Work out the finished part from the listing and answer in its coordinate system (mm). A direction names the side the tool comes from. Round coordinates to 2 decimals unless told otherwise and drop trailing zeros. Loops run counter-clockwise (first coordinate to the right, second up) from the corner with the lowest first, then second, coordinate; pieces in that order, holes last. Notation, with made-up numbers: (86.5, 5.25) -> (139.5, 5.25) arc R21 ccw to (139.5, 29.25) -> close; hole circle Ø6 at (-15, 56.5). An arc over 180 degrees is marked (long way). Use one line per item in the form item = value.
```python
from build123d import *

# Parameters (mm, degrees)
SKETCH_1_W          = 50
SKETCH_1_H          = 150
EXTRUDE_1_DEPTH     = 40
CHAMFER_1_SIZE      = 30
CHAMFER_1_SIZE2     = 60
FILLET_1_R          = 10
SKETCH_2_R          = 10
CUT_EXTRUDE_1_DEPTH = 15
CHAMFER_2_SIZE      = 1
SKETCH_3_R          = 5
CUT_EXTRUDE_2_DEPTH = 26


with BuildPart() as part:
    # 草图1 → 凸台-拉伸1 (new body)
    with BuildSketch(Plane.XY):
        with Locations((25, 75)):
            Rectangle(SKETCH_1_W, SKETCH_1_H)
    extrude(amount=EXTRUDE_1_DEPTH)

    # 倒角1
    chamfer_1_edges = [part.edges().sort_by_distance(p)[0] for p in [
        (25, 0, 40),
    ]]
    chamfer_1_side = [part.faces().sort_by_distance(p)[0] for p in [
        (25, 0, 20),
    ]]
    chamfer(chamfer_1_edges, length=CHAMFER_1_SIZE, length2=CHAMFER_1_SIZE2, reference=chamfer_1_side[0])

    # 圆角1
    fillet_1_edges = [part.edges().sort_by_distance(p)[0] for p in [
        (25, 60, 40),
    ]]
    fillet(fillet_1_edges, radius=FILLET_1_R)

    # 草图2 → 切除-拉伸1 (cut)
    with BuildSketch(Plane.XY.offset(40)):
        with Locations((25, 130)):
            Circle(SKETCH_2_R)
        with Locations((25, 80)):
            Circle(SKETCH_2_R)
    extrude(amount=-CUT_EXTRUDE_1_DEPTH, mode=Mode.SUBTRACT)

    # 倒角2
    chamfer_2_edges = [part.edges().sort_by_distance(p)[0] for p in [
        (15, 130, 40),
        (15, 80, 40),
    ]]
    chamfer(chamfer_2_edges, length=CHAMFER_2_SIZE)

    # 草图3 → 切除-拉伸2 (cut, through all)
    with BuildSketch(Plane.XY.offset(25)):
        with Locations((25, 130)):
            Circle(SKETCH_3_R)
        with Locations((25, 80)):
            Circle(SKETCH_3_R)
    extrude(amount=-CUT_EXTRUDE_2_DEPTH, mode=Mode.SUBTRACT)


solid = part.part
```
(1) Given P1, Ø10, axis at x = 20.5, z = 12, coming from the -Y side; P2, Ø16, axis at x = 25, y = 130, coming from the +Z side; P3, Ø9, axis at x = 25, y = 130, coming from the +Z side; P4, Ø1, axis at x = 6.5, z = 23.5, coming from the -Y side, each flat-ended and moving along its own axis, determine where each tip first touches the part or whether it passes through.
Completed:
P1 = 0
P2 = 25
P3 = through
P4 = 26
(2) For a pull along X with two mould halves and no side action, classify faces 1 (the cylindrical face through (20, 130, 13)), 2 (the flat face through (24.65, 29.349, 24.675)), 3 (the flat face through (50, 91, 20)) as +X half, -X half, draft (parallel to the pull), parting line (faces both ways), or undercut.
Completed:
face_1 = undercut
face_2 = draft
face_3 = +X half
(3) Find section B-B, the plane y = 130. Write down the section's boundary in (x, z).
Completed:
outline = (0, 0) -> (20, 0) -> (20, 25) -> (15, 25) -> (15, 39) -> (14, 40) -> (0, 40) -> close; (30, 0) -> (50, 0) -> (50, 40) -> (36, 40) -> (35, 39) -> (35, 25) -> (30, 25) -> close
(4) Find section D-D, the plane x = 7. Write down the section's boundary in (y, z), then the cut area to 3 significant figures.
Completed:
outline = (0, 0) -> (150, 0) -> (150, 40) -> (62.36, 40) arc R10 ccw to (57.89, 38.94) -> (0, 10) -> close
area = 5,100 mm2
(5) For faces 4 (the cylindrical face through (25.35, 60.032, 39.725)), 5 (the cylindrical face through (30.38, 88.43, 32.1)), determine the directions among +Z, -Z, +X, -X, +Y, -Y from which every point of the face is accessible in a straight line to the end or side of a thin tool.
Completed:
face_4 = +Z, +X, -X, -Y
face_5 = +Z
(6) Find section C-C, the plane z = 11.5. Write down the section's boundary in (x, y), then the cut area to 3 significant figures.
Completed:
outline = (0, 3) -> (50, 3) -> (50, 150) -> (0, 150) -> close; hole circle Ø10 at (25, 80); hole circle Ø10 at (25, 130)
area = 7,190 mm2
(7) Find section A-A, the plane x = 25. Write down the section's boundary in (y, z).
Completed:
outline = (0, 0) -> (75, 0) -> (75, 25) -> (70, 25) -> (70, 39) -> (69, 40) -> (62.36, 40) arc R10 ccw to (57.89, 38.94) -> (0, 10) -> close; (85, 0) -> (125, 0) -> (125, 25) -> (120, 25) -> (120, 39) -> (119, 40) -> (91, 40) -> (90, 39) -> (90, 25) -> (85, 25) -> close; (135, 0) -> (150, 0) -> (150, 40) -> (141, 40) -> (140, 39) -> (140, 25) -> (135, 25) -> close
(8) Consider L1, parallel to Y at x = 24, z = 27.5; L2, parallel to Y at x = 25, z = 30; L3, parallel to Z at x = 43.5, y = 27. Determine where each line is inside the solid, lowest interval first.
Completed:
L1 = 35 to 70.05, 89.95 to 120.05, 139.95 to 150
L2 = 40 to 70, 90 to 120, 140 to 150
L3 = 0 to 23.5
